Check sheet for the modelled part. Datum: model origin and axes. Units: mm. A direction names the side the tool comes from. Give positions to 0.01 mm unless a question says otherwise; leave off trailing zeros. Loops run counter-clockwise (first coordinate to the right, second up) from the corner with the lowest first, then second, coordinate; pieces in that order, holes last. Notation, with made-up numbers: (86, -10) - (100, -10) arc R22 ccw to (100, 13) - close; hole circle Ø6 at (20.25, 34.25). An arc over 180 degrees is marked (long way). Use one line per item in the form item = value.
from build123d import *

# Parameters (mm, degrees)
F0_R     = 3.96875
F0_R_2   = 1.2
F1_DEPTH = 7.62
F2_R     = 5.08


with BuildPart() as f1:
    # F0 (on Top) → F1 (new body)
    with BuildSketch(Plane.XY):
        Polygon((14.76375, 19.05), (-14.76375, 19.05), (-14.76375, 12.7), (-14.76375, -12.7), (-14.76375, -19.05), (14.76375, -19.05), (14.76375, -12.7), (47.14875, -12.7), (47.14875, 12.7), (14.76375, 12.7), align=None)
        with Locations((-3.302, -10.16)):
            Circle(F0_R, mode=Mode.SUBTRACT)
        with Locations((39.21125, -7.62)):
            Circle(F0_R_2, mode=Mode.SUBTRACT)
        with Locations((-3.302, 10.16)):
            Circle(F0_R, mode=Mode.SUBTRACT)
        with Locations((39.21125, 7.62)):
            Circle(F0_R_2, mode=Mode.SUBTRACT)
    extrude(amount=F1_DEPTH)

    # F2
    f2_edges = [f1.edges().sort_by_distance(p)[0] for p in [
        (14.76375, -12.7, 3.81),
        (14.76375, 12.7, 3.81),
    ]]
    fillet(f2_edges, radius=F2_R)


solid = f1.part
Item 1: Gauge pin test, flat ends, axial feed: P1, Ø4, axis at x = 31.5, z = 2, coming from the -Y side; P2, Ø1, axis at y = 18.5, z = 4, coming from the +X side; P3, Ø1, axis at x = -2, y = 8, coming from the +Z side; P4, Ø4, axis at x = 19.5, z = 5.5, coming from the -Y side. Record the tip position at first contact, or that the pin passes through.
Answer block:
P1 = -12.7
P2 = 14.76
P3 = through
P4 = -13.27
Item 2: Section check C-C on x = -1. Record the boundary of the cut face in (y, z), then the cut area to 3 significant figures.
Answer block:
outline = (-19.05, 0) - (-13.39, 0) - (-13.39, 7.62) - (-19.05, 7.62) - close; (-6.93, 0) - (6.93, 0) - (6.93, 7.62) - (-6.93, 7.62) - close; (13.39, 0) - (19.05, 0) - (19.05, 7.62) - (13.39, 7.62) - close
area = 192 mm2
Item 3: Access from +Z, -Z, +X, -X, +Y, -Y to the whole of each face (thin tool, end or side, straight path). Record for faces 4 (the face through (34, 12.7, 4)), 5 (the face through (-6.451, 7.745, 3.757)), 6 (the face through (14.764, -18, 4)).
Answer block:
face_4 = +Z, -Z, +X, +Y
face_5 = +Z, -Z
face_6 = +Z, -Z, +X, -Y
Item 4: Thickness scan on L1, parallel to Y at x = -3, z = 6; L2, parallel to Y at x = 39.5, z = 7.5; L3, parallel to Y at x = 19.5, z = 2.75. Record the ranges inside material, lowest first.
Answer block:
L1 = -19.05 to -14.12, -6.2 to 6.2, 14.12 to 19.05
L2 = -12.7 to -8.78, -6.46 to 6.46, 8.78 to 12.7
L3 = -12.71 to 12.71
Item 5: Section check B-B on z = 4.75. Record the boundary of the cut face in (x, y).
Answer block:
outline = (-14.76, -19.05) - (14.76, -19.05) - (14.76, -17.78) arc R5.08 cw to (19.84, -12.7) - (47.15, -12.7) - (47.15, 12.7) - (19.84, 12.7) arc R5.08 cw to (14.76, 17.78) - (14.76, 19.05) - (-14.76, 19.05) - close; hole circle Ø7.94 at (-3.3, -10.16); hole circle Ø7.94 at (-3.3, 10.16); hole circle Ø2.4 at (39.21, -7.62); hole circle Ø2.4 at (39.21, 7.62)
Item 6: Section check D-D on y = 13.5. Record the boundary of the cut face in (x, z), then the cut area to 3 significant figures.
Answer block:
outline = (-14.76, 0) - (-5.45, 0) - (-5.45, 7.62) - (-14.76, 7.62) - close; (-1.16, 0) - (17.11, 0) - (17.11, 7.62) - (-1.16, 7.62) - close
area = 210 mm2
Item 7: Mould release check, pull along X, two halves, no side actions. Record for faces 1 (the face through (16.21, 14.23, 3.86)), 2 (the face through (33, -12.7, 4)), 3 (the face through (38.012, -7.567, 3.757)): released by +X, released by -X, zero draft, split by the parting line, or undercut.
Answer block:
face_1 = released by +X
face_2 = zero draft
face_3 = undercut
Item 8: Section check A-A on y = -10.16. Record the boundary of the cut face in (x, z), then the cut area to 3 significant figures.
Answer block:
outline = (-14.76, 0) - (-7.27, 0) - (-7.27, 7.62) - (-14.76, 7.62) - close; (0.67, 0) - (47.15, 0) - (47.15, 7.62) - (0.67, 7.62) - close
area = 411 mm2
